```python
from build123d import *

# Parameters (mm, degrees)
F0_W     = 304.8
F0_H     = 57.15
F1_DEPTH = 19.05
F3_DEPTH = 6.35
F4_W     = 285.3944
F4_H     = 20.701
F5_DEPTH = 3.175
F6_W     = 85.725
F6_H     = 6.35
F7_DEPTH = 19.05


with BuildPart() as f1:
    # F0 (on Right) → F1 (new body)
    with BuildSketch(Plane.YZ):
        Rectangle(F0_W, F0_H)
    extrude(amount=F1_DEPTH)

    # F2 (on face) → F3 (cut)
    with BuildSketch(Plane.YZ.offset(19.05)):
        with BuildLine():
            ThreePointArc((146.05, 15.24), (142.6972, 18.5928), (139.3444, 15.24))
            Line((139.3444, 15.24), (139.3444, -15.2273))
            ThreePointArc((139.3444, -15.2273), (142.6972, -18.5801), (146.05, -15.2273))
            Line((146.05, -15.2273), (146.05, 15.24))
        make_face()
    extrude(amount=-F3_DEPTH, mode=Mode.SUBTRACT)

    # F4 (on face) → F5 (cut)
    with BuildSketch(Plane.YZ.offset(19.05)):
        with Locations((-3.3528, 0.8255)):
            Rectangle(F4_W, F4_H)
    extrude(amount=-F5_DEPTH, mode=Mode.SUBTRACT)

    # F6 (on face) → F7 (cut, through all)
    with BuildSketch(Plane.YZ.offset(19.05)):
        with Locations((-1.5875, 25.4)):
            Rectangle(F6_W, F6_H)
    extrude(amount=-F7_DEPTH, mode=Mode.SUBTRACT)


solid = f1.part
```
CAD build for the part. Positions are in the model's coordinates, mm. A direction names the side the tool comes from. Coordinates: 2 decimals unless noted, no trailing zeros. Order: outer loops, then holes, each group sorted by start corner. A loop starts at its lowest first (then second) coordinate and runs counter-clockwise, first axis right, second up. Notation, with made-up numbers: (20, 70.25) -> (77, 70.25) arc R21 ccw to (77, 98.25) -> close; hole circle Ø3 at (75, 9). An arc over 180 degrees is marked (long way). Use one line per item in the form item = value. Start each with the question number.
1) Band-saw the part on C-C on z = -1. Give the cut face in (x, y) (3 decimals), then the cut area to 3 significant figures.
2) Band-saw the part on B-B on y = 104. Give the cut face in (x, z) (3 decimals), then the cut area to 3 significant figures.
3) Tool access for faces 4 (the flat face through (10, 41.275, 25)), 5 (the cylindrical face through (15.92, 142.62, -18.58)), 6 (the flat face through (9, -2, -28.575)): list every direction of +Z, -Z, +X, -X, +Y, -Y with a clear straight run to the whole face (end or side of a thin tool).
4) Band-saw the part on A-A on x = 8. Give the cut face in (y, z) (3 decimals), then the cut area to 3 significant figures.
5) Drop flat-ended pins along their axis: pin 1 (1 mm diameter, centred on x = 11, y = -26, fed in from +Z) (3 decimals); pin 2 (6 mm diameter, centred on y = -48.5, z = 5, fed in from +X) (3 decimals); pin 3 (6 mm diameter, centred on y = 76.5, z = 9.5, fed in from +X). Give the stop position or say it passes through.
6) Drill centre lines: L1, parallel to Z at x = 17.75, y = -99 (3 decimals); L2, parallel to Y at x = 3, z = 23 (3 decimals); L3, parallel to Y at x = 15, z = -14.5. Where is each one in solid material? Low to high. Write a range as [from, to].
7) Pull direction Y, two halves, no side cores. Call faces 1 (the flat face through (10, -44.45, 25)), 2 (the flat face through (9, 96, 28.575)), 3 (the flat face through (9, 152.4, 0)): +Y half, -Y half, draft (parallel to the pull), parting line (faces both ways), or undercut.
Entries:
q1.outline = (0, -152.4) -> (19.05, -152.4) -> (19.05, -146.05) -> (15.875, -146.05) -> (15.875, 139.344) -> (12.7, 139.344) -> (12.7, 146.05) -> (19.05, 146.05) -> (19.05, 152.4) -> (0, 152.4) -> close
q1.area = 4,860 mm2
q2.outline = (0, -28.575) -> (19.05, -28.575) -> (19.05, -9.525) -> (15.875, -9.525) -> (15.875, 11.176) -> (19.05, 11.176) -> (19.05, 28.575) -> (0, 28.575) -> close
q2.area = 1,020 mm2
q3.face_4 = +Z, +X, -X
q3.face_5 = +X
q3.face_6 = -Z, +X, -X, +Y, -Y
q4.outline = (-152.4, -28.575) -> (152.4, -28.575) -> (152.4, 28.575) -> (41.275, 28.575) -> (41.275, 22.225) -> (-44.45, 22.225) -> (-44.45, 28.575) -> (-152.4, 28.575) -> close
q4.area = 16,900 mm2
q5.pin_1 = 22.225
q5.pin_2 = 15.875
q5.pin_3 = 19.05
q6.L1 = [-28.575, -9.525], [11.176, 28.575]
q6.L2 = [-152.4, -44.45], [41.275, 152.4]
q6.L3 = [-152.4, 139.34], [146.05, 152.4]
q7.face_1 = undercut
q7.face_2 = draft
q7.face_3 = +Y half
